The listing builds one solid part. Answer for the finished solid, in the listing's coordinates (mm). A direction names the side the tool comes from. Round coordinates to 2 decimals unless told otherwise and drop trailing zeros. Write each loop counter-clockwise with the first axis right and the second up, starting at its lowest first coordinate (ties: lowest second). Pieces come first, ordered by that corner, then holes.
Item 1: For a pull along Z with two mould halves and no side action, classify faces 4 (the face through (34.292, 38.712, -11.352)), 5 (the face through (18.66, 42.49, -6.76)), 6 (the face through (45, 43, -10)) as +Z half, -Z half, draft (parallel to the pull), parting line (faces both ways), or undercut.
Item 2: Each of these flat-tipped pins is pushed along its axis until it touches: pin 1 (2 mm diameter, centred on y = 38.5, z = -19, fed in from +X); pin 2 (3 mm diameter, centred on x = 42.5, y = 27.5, fed in from +Z); pin 3 (2 mm diameter, centred on x = -4.5, z = -13.5, fed in from +Y); pin 4 (6.5 mm diameter, centred on x = 45, z = -5, fed in from -Y). Where does it stop, or does it pass through?
Item 3: Find section A-A on x = -5. Give the vertices of the cut face in (y, z).
Item 4: A tool of negligible diameter and unlimited length cuts with its end or side. For faces 1 (the face through (17, 43, -10)), 2 (the face through (43, 27, -19)), 3 (the face through (0, 13, -10)), from which of +Z, -Z, +X, -X, +Y, -Y can it reach the whole face along a straight path? Write none if from no direction.
Item 5: Find section C-C on x = 2.5. Give the vertices of the cut face in (y, z).
Item 6: Find section D-D on y = 13. Give the vertices of the cut face in (x, z).
Item 7: Find the intervals of material crossed by probe 1 along Y at (x, z) = (27.5, -6); probe 2 along Z at (x, y) = (19, 15); probe 3 along Y at (x, z) = (43, -2.5), in increasing order.
Item 8: Find section B-B on z = 4. Give the vertices of the cut face in (x, y), then the cut area to 3 significant figures.
```python
from build123d import *

# Parameters (mm, degrees)
SKETCH2_W           = 40
SKETCH2_H           = 20
BOSS_EXTRUDE1_DEPTH = 36
FILLET1_R           = 1
SKETCH4_W           = 18
SKETCH4_H           = 2.5
BOSS_EXTRUDE2_DEPTH = 7
CUT_EXTRUDE1_REACH  = 30.5
SKETCH5_R           = 2.5
FILLET2_R           = 1
SKETCH7_W           = 18
SKETCH7_H           = 2.5
BOSS_EXTRUDE3_DEPTH = 7
FILLET3_R           = 1
CUT_EXTRUDE2_REACH  = 30.5
SKETCH8_R           = 2.5
SKETCH9_R           = 4.5
BOSS_EXTRUDE4_DEPTH = 5.5
BOSS_EXTRUDE5_DEPTH = 2
CUT_EXTRUDE3_REACH  = 45.5
SKETCH11_R          = 1
SKETCH12_W          = 6
SKETCH12_H          = 3
BOSS_EXTRUDE6_DEPTH = 7


with BuildPart() as part:
    # Sketch2 → Boss-Extrude1 (new body)
    with BuildSketch(Plane(origin=(0, 0, 0), x_dir=(1, 0, 0), z_dir=(0, 1, 0))):
        with Locations((20, 10)):
            Rectangle(SKETCH2_W, SKETCH2_H)
    extrude(amount=BOSS_EXTRUDE1_DEPTH)

    # Fillet1
    fillet1_edges = [part.edges().sort_by_distance(p)[0] for p in [
        (40, 36, -10),
        (20, 36, -20),
        (0, 36, -10),
        (20, 0, -20),
        (40, 0, -10),
        (20, 0, 0),
        (0, 0, -10),
        (20, 36, 0),
        (0, 18, -20),
        (40, 18, -20),
        (40, 18, 0),
        (0, 18, 0),
    ]]
    fillet(fillet1_edges, radius=FILLET1_R)

    # Sketch4 → Boss-Extrude2 (add)
    with BuildSketch(Plane(origin=(40, 0, 0), x_dir=(0, 0, -1), z_dir=(1, 0, 0))):
        with Locations((10, 27.25)):
            Rectangle(SKETCH4_W, SKETCH4_H)
    extrude(amount=BOSS_EXTRUDE2_DEPTH)

    # Sketch5 → Cut-Extrude1 (cut, up to next)
    with BuildSketch(Plane(origin=(0, 28.5, 0), x_dir=(1, 0, 0), z_dir=(0, 1, 0)), mode=Mode.PRIVATE) as cut_extrude1_sk1:
        with Locations((45, 5)):
            Circle(SKETCH5_R)
    cut_extrude1_tool1 = extrude(cut_extrude1_sk1.sketch, amount=-CUT_EXTRUDE1_REACH, mode=Mode.PRIVATE) & part.part
    add(cut_extrude1_tool1.solids().sort_by_distance((45, 28.5, -5))[0], mode=Mode.SUBTRACT)
    # Sketch5 → Cut-Extrude1 (cut, up to next)
    with BuildSketch(Plane(origin=(0, 28.5, 0), x_dir=(1, 0, 0), z_dir=(0, 1, 0)), mode=Mode.PRIVATE) as cut_extrude1_sk2:
        with Locations((45, 15)):
            Circle(SKETCH5_R)
    cut_extrude1_tool2 = extrude(cut_extrude1_sk2.sketch, amount=-CUT_EXTRUDE1_REACH, mode=Mode.PRIVATE) & part.part
    add(cut_extrude1_tool2.solids().sort_by_distance((45, 28.5, -15))[0], mode=Mode.SUBTRACT)

    # Fillet2
    fillet2_edges = [part.edges().sort_by_distance(p)[0] for p in [
        (47, 27.25, -19),
        (47, 27.25, -1),
    ]]
    fillet(fillet2_edges, radius=FILLET2_R)

    # Sketch7 → Boss-Extrude3 (add)
    with BuildSketch(Plane.ZY):
        with Locations((-10, 27.25)):
            Rectangle(SKETCH7_W, SKETCH7_H)
    extrude(amount=BOSS_EXTRUDE3_DEPTH)

    # Fillet3
    fillet3_edges = [part.edges().sort_by_distance(p)[0] for p in [
        (-7, 27.25, -19),
        (-7, 27.25, -1),
    ]]
    fillet(fillet3_edges, radius=FILLET3_R)

    # Sketch8 → Cut-Extrude2 (cut, up to next)
    with BuildSketch(Plane(origin=(0, 28.5, 0), x_dir=(1, 0, 0), z_dir=(0, 1, 0)), mode=Mode.PRIVATE) as cut_extrude2_sk1:
        with Locations((-5, 15)):
            Circle(SKETCH8_R)
    cut_extrude2_tool1 = extrude(cut_extrude2_sk1.sketch, amount=-CUT_EXTRUDE2_REACH, mode=Mode.PRIVATE) & part.part
    add(cut_extrude2_tool1.solids().sort_by_distance((-5, 28.5, -15))[0], mode=Mode.SUBTRACT)
    # Sketch8 → Cut-Extrude2 (cut, up to next)
    with BuildSketch(Plane(origin=(0, 28.5, 0), x_dir=(1, 0, 0), z_dir=(0, 1, 0)), mode=Mode.PRIVATE) as cut_extrude2_sk2:
        with Locations((-5, 5)):
            Circle(SKETCH8_R)
    cut_extrude2_tool2 = extrude(cut_extrude2_sk2.sketch, amount=-CUT_EXTRUDE2_REACH, mode=Mode.PRIVATE) & part.part
    add(cut_extrude2_tool2.solids().sort_by_distance((-5, 28.5, -5))[0], mode=Mode.SUBTRACT)

    # Sketch9 → Boss-Extrude4 (add)
    with BuildSketch(Plane(origin=(0, 36, 0), x_dir=(1, 0, 0), z_dir=(0, 1, 0))):
        with Locations((30, 10)):
            Circle(SKETCH9_R)
    extrude(amount=BOSS_EXTRUDE4_DEPTH)

    # Sketch10 → Boss-Extrude5 (add)
    with BuildSketch(Plane(origin=(0, 41.5, 0), x_dir=(1, 0, 0), z_dir=(0, 1, 0))):
        with BuildLine():
            Line((27.5, 27.5), (26, 15))
            ThreePointArc((26, 15), (25.672931537, 14.327068463), (25, 14))
            Line((25, 14), (12.5, 12.5))
            ThreePointArc((12.5, 12.5), (10.817671157, 11.682328843), (10, 10))
            ThreePointArc((10, 10), (10.817671157, 8.317671157), (12.5, 7.5))
            Line((12.5, 7.5), (25, 6))
            ThreePointArc((25, 6), (25.707106781, 5.707106781), (26, 5))
            Line((26, 5), (27.5, -7.5))
            ThreePointArc((27.5, -7.5), (28.317671157, -9.182328843), (30, -10))
            ThreePointArc((30, -10), (31.682328843, -9.182328843), (32.5, -7.5))
            Line((32.5, -7.5), (34, 5))
            ThreePointArc((34, 5), (34.292893219, 5.707106781), (35, 6))
            Line((35, 6), (47.5, 7.5))
            ThreePointArc((47.5, 7.5), (49.182328843, 8.317671157), (50, 10))
            ThreePointArc((50, 10), (49.182328843, 11.682328843), (47.5, 12.5))
            Line((47.5, 12.5), (35, 14))
            ThreePointArc((35, 14), (34.292893219, 14.292893219), (34, 15))
            Line((34, 15), (32.5, 27.5))
            ThreePointArc((32.5, 27.5), (31.682328843, 29.182328843), (30, 30))
            ThreePointArc((30, 30), (28.317671157, 29.182328843), (27.5, 27.5))
        make_face()
    extrude(amount=BOSS_EXTRUDE5_DEPTH)

    # Sketch11 → Cut-Extrude3 (cut, up to next)
    with BuildSketch(Plane(origin=(0, 43.5, 0), x_dir=(1, 0, 0), z_dir=(0, 1, 0)), mode=Mode.PRIVATE) as cut_extrude3_sk1:
        with Locations((30, 27)):
            Circle(SKETCH11_R)
    cut_extrude3_tool1 = extrude(cut_extrude3_sk1.sketch, amount=-CUT_EXTRUDE3_REACH, mode=Mode.PRIVATE) & part.part
    add(cut_extrude3_tool1.solids().sort_by_distance((30, 43.5, -27))[0], mode=Mode.SUBTRACT)
    # Sketch11 → Cut-Extrude3 (cut, up to next)
    with BuildSketch(Plane(origin=(0, 43.5, 0), x_dir=(1, 0, 0), z_dir=(0, 1, 0)), mode=Mode.PRIVATE) as cut_extrude3_sk2:
        with Locations((30, 24)):
            Circle(SKETCH11_R)
    cut_extrude3_tool2 = extrude(cut_extrude3_sk2.sketch, amount=-CUT_EXTRUDE3_REACH, mode=Mode.PRIVATE) & part.part
    add(cut_extrude3_tool2.solids().sort_by_distance((30, 43.5, -24))[0], mode=Mode.SUBTRACT)
    # Sketch11 → Cut-Extrude3 (cut, up to next)
    with BuildSketch(Plane(origin=(0, 43.5, 0), x_dir=(1, 0, 0), z_dir=(0, 1, 0)), mode=Mode.PRIVATE) as cut_extrude3_sk3:
        with Locations((30, 21)):
            Circle(SKETCH11_R)
    cut_extrude3_tool3 = extrude(cut_extrude3_sk3.sketch, amount=-CUT_EXTRUDE3_REACH, mode=Mode.PRIVATE) & part.part
    add(cut_extrude3_tool3.solids().sort_by_distance((30, 43.5, -21))[0], mode=Mode.SUBTRACT)
    # Sketch11 → Cut-Extrude3 (cut, up to next)
    with BuildSketch(Plane(origin=(0, 43.5, 0), x_dir=(1, 0, 0), z_dir=(0, 1, 0)), mode=Mode.PRIVATE) as cut_extrude3_sk4:
        with Locations((30, 18)):
            Circle(SKETCH11_R)
    cut_extrude3_tool4 = extrude(cut_extrude3_sk4.sketch, amount=-CUT_EXTRUDE3_REACH, mode=Mode.PRIVATE) & part.part
    add(cut_extrude3_tool4.solids().sort_by_distance((30, 43.5, -18))[0], mode=Mode.SUBTRACT)
    # Sketch11 → Cut-Extrude3 (cut, up to next)
    with BuildSketch(Plane(origin=(0, 43.5, 0), x_dir=(1, 0, 0), z_dir=(0, 1, 0)), mode=Mode.PRIVATE) as cut_extrude3_sk5:
        with Locations((47, 10)):
            Circle(SKETCH11_R)
    cut_extrude3_tool5 = extrude(cut_extrude3_sk5.sketch, amount=-CUT_EXTRUDE3_REACH, mode=Mode.PRIVATE) & part.part
    add(cut_extrude3_tool5.solids().sort_by_distance((47, 43.5, -10))[0], mode=Mode.SUBTRACT)
    # Sketch11 → Cut-Extrude3 (cut, up to next)
    with BuildSketch(Plane(origin=(0, 43.5, 0), x_dir=(1, 0, 0), z_dir=(0, 1, 0)), mode=Mode.PRIVATE) as cut_extrude3_sk6:
        with Locations((44, 10)):
            Circle(SKETCH11_R)
    cut_extrude3_tool6 = extrude(cut_extrude3_sk6.sketch, amount=-CUT_EXTRUDE3_REACH, mode=Mode.PRIVATE) & part.part
    add(cut_extrude3_tool6.solids().sort_by_distance((44, 43.5, -10))[0], mode=Mode.SUBTRACT)
    # Sketch11 → Cut-Extrude3 (cut, up to next)
    with BuildSketch(Plane(origin=(0, 43.5, 0), x_dir=(1, 0, 0), z_dir=(0, 1, 0)), mode=Mode.PRIVATE) as cut_extrude3_sk7:
        with Locations((41, 10)):
            Circle(SKETCH11_R)
    cut_extrude3_tool7 = extrude(cut_extrude3_sk7.sketch, amount=-CUT_EXTRUDE3_REACH, mode=Mode.PRIVATE) & part.part
    add(cut_extrude3_tool7.solids().sort_by_distance((41, 43.5, -10))[0], mode=Mode.SUBTRACT)
    # Sketch11 → Cut-Extrude3 (cut, up to next)
    with BuildSketch(Plane(origin=(0, 43.5, 0), x_dir=(1, 0, 0), z_dir=(0, 1, 0)), mode=Mode.PRIVATE) as cut_extrude3_sk8:
        with Locations((38, 10)):
            Circle(SKETCH11_R)
    cut_extrude3_tool8 = extrude(cut_extrude3_sk8.sketch, amount=-CUT_EXTRUDE3_REACH, mode=Mode.PRIVATE) & part.part
    add(cut_extrude3_tool8.solids().sort_by_distance((38, 43.5, -10))[0], mode=Mode.SUBTRACT)
    # Sketch11 → Cut-Extrude3 (cut, up to next)
    with BuildSketch(Plane(origin=(0, 43.5, 0), x_dir=(1, 0, 0), z_dir=(0, 1, 0)), mode=Mode.PRIVATE) as cut_extrude3_sk9:
        with Locations((30, -7)):
            Circle(SKETCH11_R)
    cut_extrude3_tool9 = extrude(cut_extrude3_sk9.sketch, amount=-CUT_EXTRUDE3_REACH, mode=Mode.PRIVATE) & part.part
    add(cut_extrude3_tool9.solids().sort_by_distance((30, 43.5, 7))[0], mode=Mode.SUBTRACT)
    # Sketch11 → Cut-Extrude3 (cut, up to next)
    with BuildSketch(Plane(origin=(0, 43.5, 0), x_dir=(1, 0, 0), z_dir=(0, 1, 0)), mode=Mode.PRIVATE) as cut_extrude3_sk10:
        with Locations((30, -4)):
            Circle(SKETCH11_R)
    cut_extrude3_tool10 = extrude(cut_extrude3_sk10.sketch, amount=-CUT_EXTRUDE3_REACH, mode=Mode.PRIVATE) & part.part
    add(cut_extrude3_tool10.solids().sort_by_distance((30, 43.5, 4))[0], mode=Mode.SUBTRACT)
    # Sketch11 → Cut-Extrude3 (cut, up to next)
    with BuildSketch(Plane(origin=(0, 43.5, 0), x_dir=(1, 0, 0), z_dir=(0, 1, 0)), mode=Mode.PRIVATE) as cut_extrude3_sk11:
        with Locations((30, -1)):
            Circle(SKETCH11_R)
    cut_extrude3_tool11 = extrude(cut_extrude3_sk11.sketch, amount=-CUT_EXTRUDE3_REACH, mode=Mode.PRIVATE) & part.part
    add(cut_extrude3_tool11.solids().sort_by_distance((30, 43.5, 1))[0], mode=Mode.SUBTRACT)
    # Sketch11 → Cut-Extrude3 (cut, up to next)
    with BuildSketch(Plane(origin=(0, 43.5, 0), x_dir=(1, 0, 0), z_dir=(0, 1, 0)), mode=Mode.PRIVATE) as cut_extrude3_sk12:
        with Locations((30, 2)):
            Circle(SKETCH11_R)
    cut_extrude3_tool12 = extrude(cut_extrude3_sk12.sketch, amount=-CUT_EXTRUDE3_REACH, mode=Mode.PRIVATE) & part.part
    add(cut_extrude3_tool12.solids().sort_by_distance((30, 43.5, -2))[0], mode=Mode.SUBTRACT)
    # Sketch11 → Cut-Extrude3 (cut, up to next)
    with BuildSketch(Plane(origin=(0, 43.5, 0), x_dir=(1, 0, 0), z_dir=(0, 1, 0)), mode=Mode.PRIVATE) as cut_extrude3_sk13:
        with Locations((13, 10)):
            Circle(SKETCH11_R)
    cut_extrude3_tool13 = extrude(cut_extrude3_sk13.sketch, amount=-CUT_EXTRUDE3_REACH, mode=Mode.PRIVATE) & part.part
    add(cut_extrude3_tool13.solids().sort_by_distance((13, 43.5, -10))[0], mode=Mode.SUBTRACT)
    # Sketch11 → Cut-Extrude3 (cut, up to next)
    with BuildSketch(Plane(origin=(0, 43.5, 0), x_dir=(1, 0, 0), z_dir=(0, 1, 0)), mode=Mode.PRIVATE) as cut_extrude3_sk14:
        with Locations((16, 10)):
            Circle(SKETCH11_R)
    cut_extrude3_tool14 = extrude(cut_extrude3_sk14.sketch, amount=-CUT_EXTRUDE3_REACH, mode=Mode.PRIVATE) & part.part
    add(cut_extrude3_tool14.solids().sort_by_distance((16, 43.5, -10))[0], mode=Mode.SUBTRACT)
    # Sketch11 → Cut-Extrude3 (cut, up to next)
    with BuildSketch(Plane(origin=(0, 43.5, 0), x_dir=(1, 0, 0), z_dir=(0, 1, 0)), mode=Mode.PRIVATE) as cut_extrude3_sk15:
        with Locations((19, 10)):
            Circle(SKETCH11_R)
    cut_extrude3_tool15 = extrude(cut_extrude3_sk15.sketch, amount=-CUT_EXTRUDE3_REACH, mode=Mode.PRIVATE) & part.part
    add(cut_extrude3_tool15.solids().sort_by_distance((19, 43.5, -10))[0], mode=Mode.SUBTRACT)
    # Sketch11 → Cut-Extrude3 (cut, up to next)
    with BuildSketch(Plane(origin=(0, 43.5, 0), x_dir=(1, 0, 0), z_dir=(0, 1, 0)), mode=Mode.PRIVATE) as cut_extrude3_sk16:
        with Locations((22, 10)):
            Circle(SKETCH11_R)
    cut_extrude3_tool16 = extrude(cut_extrude3_sk16.sketch, amount=-CUT_EXTRUDE3_REACH, mode=Mode.PRIVATE) & part.part
    add(cut_extrude3_tool16.solids().sort_by_distance((22, 43.5, -10))[0], mode=Mode.SUBTRACT)

    # Sketch12 → Boss-Extrude6 (add)
    with BuildSketch(Plane(origin=(40, 0, 0), x_dir=(0, 0, -1), z_dir=(1, 0, 0))):
        with Locations((10, 2.5)):
            Rectangle(SKETCH12_W, SKETCH12_H)
    extrude(amount=BOSS_EXTRUDE6_DEPTH)


solid = part.part
```
Check values:
1. face 4: parting line
1. face 5: +Z half
1. face 6: undercut
2. pin 1: passes through
2. pin 2: stops at z = -1
2. pin 3: stops at y = 28.5
2. pin 4: stops at y = 1
3. outline: (26, -19) - (28.5, -19) - (28.5, -17.5) - (26, -17.5) - close; (26, -12.5) - (28.5, -12.5) - (28.5, -7.5) - (26, -7.5) - close; (26, -2.5) - (28.5, -2.5) - (28.5, -1) - (26, -1) - close
4. face 1: +Y
4. face 2: -Z, +X, +Y, -Y
4. face 3: +Z, -Z, -X, -Y
5. outline: (0, -19) arc R1 ccw to (1, -20) - (35, -20) arc R1 ccw to (36, -19) - (36, -1) arc R1 ccw to (35, 0) - (1, 0) arc R1 ccw to (0, -1) - close
6. outline: (0, -19) arc R1 ccw to (1, -20) - (39, -20) arc R1 ccw to (40, -19) - (40, -1) arc R1 ccw to (39, 0) - (1, 0) arc R1 ccw to (0, -1) - close
7. probe 1: y = 0 to 36, 41.5 to 43.5
7. probe 2: z = -20 to 0
7. probe 3: y = 26 to 28.5
8. outline: (27.08, 41.5) - (29, 41.5) - (29, 43.5) - (27.08, 43.5) - close; (31, 41.5) - (32.92, 41.5) - (32.92, 43.5) - (31, 43.5) - close
8. area: 7.68 mm2
